Job drawing, mm, ordinate dimensions from the low corner. One solid piece. A direction names the side the tool comes from. Coordinates: 2 decimals unless noted, no trailing zeros. Loops run counter-clockwise (first coordinate to the right, second up) from the corner with the lowest first, then second, coordinate; pieces in that order, holes last. Notation, with made-up numbers: (82.5, 63) - (116.5, 63) arc R25 cw to (116.5, 101) - close; hole circle Ø7 at (59.25, 50). An arc over 180 degrees is marked (long way). Use a Markdown table: item, result. Add a question column.
1. Band-saw the part on D-D, the plane y = 2.25. Give the cut face in (x, z).
2. Band-saw the part on A-A, the plane x = 40. Give the cut face in (y, z), plus the area to 3 significant figures.
3. Wall check: probe 1 along X at (y, z) = (17.5, 10); probe 2 along Y at (x, z) = (62.5, 14.75); probe 3 along Z at (x, y) = (70, 2). Give the ranges that are in metal, low to high. Write a range as [from, to].
4. Drop flat-ended pins along their axis: pin 1 (1.5 mm diameter, centred on y = 9, z = 18, fed in from -X); pin 2 (8 mm diameter, centred on y = 11.5, z = 15, fed in from -X); pin 3 (7 mm diameter, centred on x = 70, z = 10, fed in from -Y); pin 4 (1 mm diameter, centred on y = 13, z = 7.5, fed in from -X). Give the stop position or say it passes through.
5. Pull direction Z, two halves, no side cores. Call the marked faces 1, 2, 3 and 4: pulls with the +Z half, pulls with the -Z half, needs draft (parallel to the pull), parting line crosses it, or undercut.
6. Band-saw the part on C-C, the plane x = 69. Give the cut face in (y, z), plus the area to 3 significant figures.
7. Band-saw the part on B-B, the plane z = 12.75. Count the separate pieces of the cut face and the enclosed holes in it, plus the area to 3 significant figures.
8. 3-axis set-ups, long thin cutter, end or side, ignore diameter. For the marked faces 5 and 6: which of +Z, -Z, +X, -X, +Y, -Y reach the whole face in a straight line?
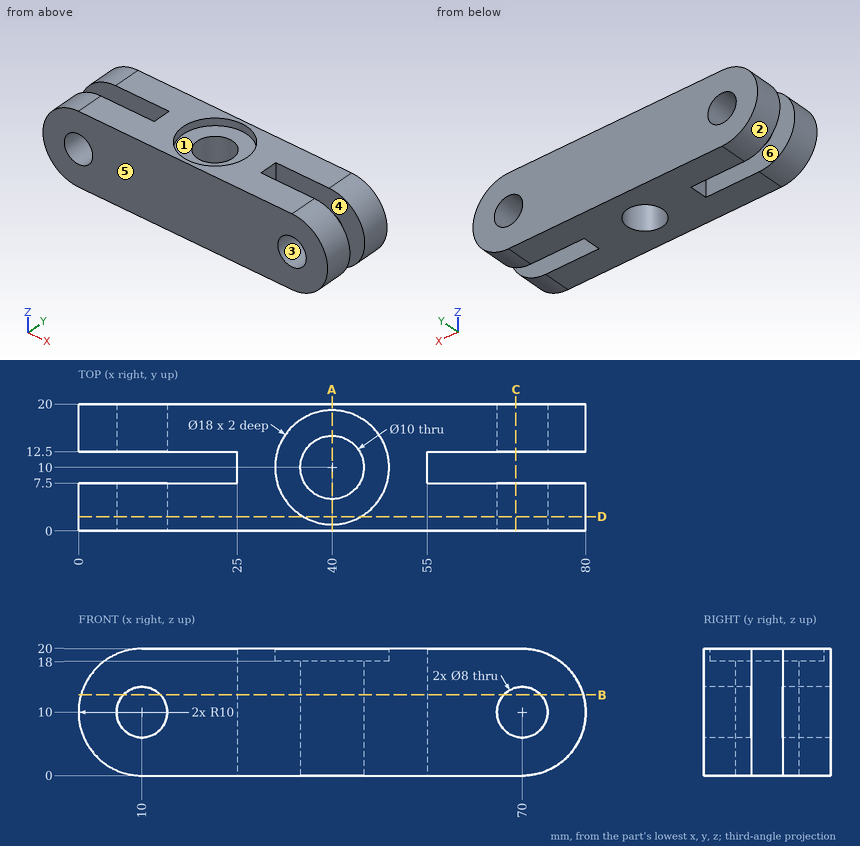
Geometry check:
| question | item | result |
|---|---|---|
| 1 | outline | (10, 0) - (70, 0) arc R10 ccw to (70, 20) - (44.58, 20) - (44.58, 18) - (35.42, 18) - (35.42, 20) - (10, 20) arc R10 ccw to start; hole circle Ø8 at (10, 10); hole circle Ø8 at (70, 10) |
| 2 | outline | (0, 0) - (5, 0) - (5, 18) - (1, 18) - (1, 20) - (0, 20) - close; (15, 0) - (20, 0) - (20, 20) - (19, 20) - (19, 18) - (15, 18) - close |
| 2 | area | 184 mm^2 |
| 3 | probe 1 | x = [0, 6], [14, 66], [74, 80] |
| 3 | probe 2 | y = [0, 7.5], [12.5, 20] |
| 3 | probe 3 | z = [0, 6], [14, 20] |
| 4 | pin 1 | stops at x = 25 |
| 4 | pin 2 | stops at x = 0.06 |
| 4 | pin 3 | passes through |
| 4 | pin 4 | stops at x = 0.2 |
| 5 | face 1 | pulls with the +Z half |
| 5 | face 2 | parting line crosses it |
| 5 | face 3 | undercut |
| 5 | face 4 | needs draft |
| 6 | outline | (0, 0) - (7.5, 0) - (7.5, 6.13) - (0, 6.13) - close; (0, 13.87) - (7.5, 13.87) - (7.5, 20) - (0, 20) - close; (12.5, 0) - (20, 0) - (20, 6.13) - (12.5, 6.13) - close; (12.5, 13.87) - (20, 13.87) - (20, 20) - (12.5, 20) - close |
| 6 | area | 184 mm^2 |
| 7 | separate pieces | 5 |
| 7 | enclosed holes | 1 |
| 7 | area | 1,090 mm^2 |
| 8 | face 5 | +Z, -Z, +X, -X, -Y |
| 8 | face 6 | +Z, -Z, -X |
